from build123d import *

# Parameters (mm, degrees)
F0_W           = 50.8
F0_H           = 38.1
F1_DEPTH       = 3.175
F3_START       = -18.288
F2_W           = 38.1
F2_H           = 69.85
F3_DEPTH       = 3.556
F5_START       = 27.686
F4_W           = 38.1
F4_H           = 69.85
F5_DEPTH       = 3.81
F6_W           = 19.05
F6_H           = 53.975
F7_DEPTH       = 32.004
F8_T1_DEPTH    = 64.9044340938
F8_T3_DEPTH    = 19.05
F8_T5_DEPTH    = 62.6934442484
F8_T11_DEPTH   = 64.9044340938
F8_T15_DEPTH   = 31.165027858
F8_T23_DEPTH   = 31.165027858
F8_T28_DEPTH   = 64.9044340938
F9_W           = 54.9304988235
F9_H           = 1.4888443984
F10_DEPTH      = 28.4988
F10_DEPTH_BACK = 25.4


# Not quite as in the source:
# - a fillet or chamfer that OpenCascade refuses, or shapes differently, is made with other operations: its cross-section is extruded or revolved along the edge and cut away or added


with BuildPart() as f1:
    # F0 (on Top) → F1 (new body)
    with BuildSketch(Plane.XY):
        with Locations((3.5055922344, 6.6658267866)):
            Rectangle(F0_W, F0_H)
    extrude(amount=F1_DEPTH)

    # F2 (on Right) → F3 (join)
    with BuildSketch(Plane.YZ.offset(F3_START)):
        with Locations((6.8596902806, -32.1689685807)):
            Rectangle(F2_W, F2_H)
    extrude(amount=-F3_DEPTH)

    # F4 (on Right) → F5 (join)
    with BuildSketch(Plane.YZ.offset(F5_START)):
        with Locations((7.2173965164, -31.5503366292)):
            Rectangle(F4_W, F4_H)
    extrude(amount=F5_DEPTH)

    # F6 (on Right) → F7 (cut)
    with BuildSketch(Plane.YZ):
        with Locations((6.4956571441, -41.2920623448)):
            Rectangle(F6_W, F6_H)
    extrude(amount=-F7_DEPTH, mode=Mode.SUBTRACT)

    # F8: fillet of radius 5.08 on 4 edges, made by hand

    # F8_s2 → F8_t1 (cut)
    with BuildSketch(Plane.XY.offset(-79.2089964387)):
        with BuildLine():
            ThreePointArc((-18.288, 20.8666682873), (-19.2723730639, 17.8612997575), (-21.844, 16.0206571441))
            Line((-21.844, 16.0206571441), (-18.288, 16.0206571441))
            Line((-18.288, 16.0206571441), (-18.288, 20.8666682873))
        make_face()
        with BuildLine():
            ThreePointArc((-18.288, -7.8753539991), (-19.2723730639, -4.8699854693), (-21.844, -3.0293428559))
            Line((-21.844, -3.0293428559), (-18.288, -3.0293428559))
            Line((-18.288, -3.0293428559), (-18.288, -7.8753539991))
        make_face()
    extrude(amount=F8_T1_DEPTH, mode=Mode.SUBTRACT)

    # F8_s4 → F8_t3 (cut)
    with BuildSketch(Plane.XZ.offset(-16.0206571441)):
        with BuildLine():
            ThreePointArc((-18.288, -9.4585512016), (-19.2723730639, -12.4639197314), (-21.844, -14.3045623448))
            Line((-21.844, -14.3045623448), (-18.288, -14.3045623448))
            Line((-18.288, -14.3045623448), (-18.288, -9.4585512016))
        make_face()
    extrude(amount=F8_T3_DEPTH, mode=Mode.SUBTRACT)

    # F8_s6 → F8_t5 (cut)
    with BuildSketch(Plane.XZ.offset(-38.5641186406)):
        with BuildLine():
            ThreePointArc((27.686, -61.5566477795), (28.7499073716, -64.6674997528), (31.496, -66.4753366292))
            Line((31.496, -66.4753366292), (27.686, -66.4753366292))
            Line((27.686, -66.4753366292), (27.686, -61.5566477795))
        make_face()
    extrude(amount=F8_T5_DEPTH, mode=Mode.SUBTRACT)


with BuildPart() as f8_tool9:
    # F8_s10 → F8_t11 (new body)
    with BuildSketch(Plane.XY.offset(-67.0939685807)):
        with BuildLine():
            ThreePointArc((-18.288, 20.8666682873), (-19.2723730639, 17.8612997575), (-21.844, 16.0206571441))
            Line((-21.844, 16.0206571441), (-18.288, 16.0206571441))
            Line((-18.288, 16.0206571441), (-18.288, 20.8666682873))
        make_face()
    extrude(amount=F8_T11_DEPTH)

    split(bisect_by=Plane.XY.offset(-14.3045623448), keep=Keep.TOP)


with BuildPart() as f8_tool13:
    # F8_s14 → F8_t15 (new body)
    with BuildSketch(Plane.XZ.offset(-28.1356850021)):
        with BuildLine():
            ThreePointArc((-18.288, -9.4585512016), (-19.2723730639, -12.4639197314), (-21.844, -14.3045623448))
            Line((-21.844, -14.3045623448), (-18.288, -14.3045623448))
            Line((-18.288, -14.3045623448), (-18.288, -9.4585512016))
        make_face()
    extrude(amount=F8_T15_DEPTH)

    split(bisect_by=Plane.XZ.offset(-25.9096902806), keep=Keep.TOP)

    split(bisect_by=Plane.XZ.offset(-16.0206571441), keep=Keep.BOTTOM)


with BuildPart() as f8_tool9_1:
    add(f8_tool9.part)

    # F8_t18: intersect F8_tool13
    add(f8_tool13.part, mode=Mode.INTERSECT)


with BuildPart() as f1_1:
    add(f1.part)

    # F8_t7: cut F8_tool9
    add(f8_tool9_1.part, mode=Mode.SUBTRACT)


with BuildPart() as f8_tool21:
    # F8_s22 → F8_t23 (new body)
    with BuildSketch(Plane.XZ.offset(-16.0206571441)):
        with BuildLine():
            ThreePointArc((-18.288, -9.4585512016), (-19.2723730639, -12.4639197314), (-21.844, -14.3045623448))
            Line((-21.844, -14.3045623448), (-18.288, -14.3045623448))
            Line((-18.288, -14.3045623448), (-18.288, -9.4585512016))
        make_face()
    extrude(amount=F8_T23_DEPTH)

    split(bisect_by=Plane.XZ.offset(12.1903097194), keep=Keep.BOTTOM)

    split(bisect_by=Plane.XZ.offset(3.0293428559), keep=Keep.TOP)


with BuildPart() as f8_tool26:
    # F8_s27 → F8_t28 (new body)
    with BuildSketch(Plane.XY.offset(-2.1895344868)):
        with BuildLine():
            ThreePointArc((-18.288, -7.8753539991), (-19.2723730639, -4.8699854693), (-21.844, -3.0293428559))
            Line((-21.844, -3.0293428559), (-18.288, -3.0293428559))
            Line((-18.288, -3.0293428559), (-18.288, -7.8753539991))
        make_face()
    extrude(amount=-F8_T28_DEPTH)

    split(bisect_by=Plane.XY.offset(-14.3045623448), keep=Keep.TOP)


with BuildPart() as f8_tool21_1:
    add(f8_tool21.part)

    # F8_t30: intersect F8_tool26
    add(f8_tool26.part, mode=Mode.INTERSECT)


with BuildPart() as f1_2:
    add(f1_1.part)

    # F8_t19: cut F8_tool21
    add(f8_tool21_1.part, mode=Mode.SUBTRACT)

    # F9 (on Front) → F10 (cut, two sides)
    with BuildSketch(Plane.XZ) as f10_sk:
        with Locations((4.6410532668, 3.4134599846)):
            Rectangle(F9_W, F9_H)
    extrude(amount=-F10_DEPTH, mode=Mode.SUBTRACT)
    extrude(f10_sk.sketch, amount=F10_DEPTH_BACK, mode=Mode.SUBTRACT)


solid = f1_2.part
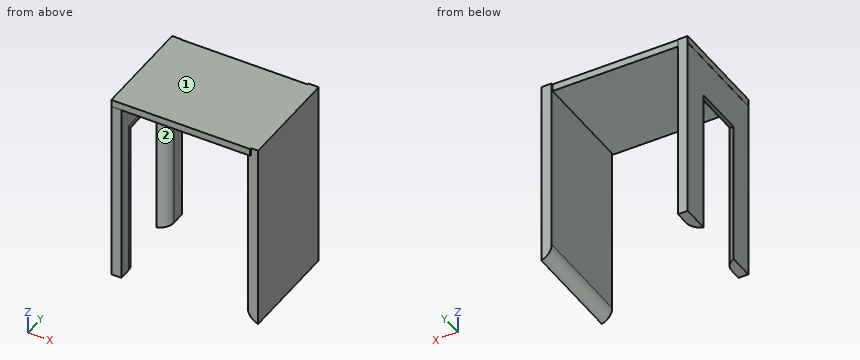
CAD build for the part. Positions are in the model's coordinates, mm. Face numbers are marked on the shaded views. Give positions to 0.01 mm unless a question says otherwise; leave off trailing zeros. Write each loop counter-clockwise with the first axis right and the second up, starting at its lowest first coordinate (ties: lowest second). Pieces come first, ordered by that corner, then holes. Notation, with made-up numbers: M 6.5,46.5 L 10.5,46.5 A23 cw 10.5,58.5 Z; hole C -13.5,61.25 d1. An arc over 180 degrees is marked long. Put each result on its own line as item: value. Start each with the question number.
(1) Band-saw the part on D-D, the plane x = -10.5. Write the cut outline in (y, z), and give its area (3 significant figures).
(2) Band-saw the part on B-B, the plane z = -38.5. Write the cut outline in (x, y).
(3) Band-saw the part on C-C, the plane y = 14. Write the cut outline in (x, z).
(4) Band-saw the part on A-A, the plane z = -2. Write the cut outline in (x, y).
(5) Probe L1, parallel to X at y = 18, z = -5; L2, parallel to X at y = 13, z = -51; L3, parallel to Z at x = -13, y = 15.5. List the from-to ranges inside material, lowest first.
(6) Mould opens along Y. For the marked faces 1 and 2 say: +Y half, -Y half, draft (parallel to the pull), parting line (faces both ways), or undercut.
(7) Flat gauge pins, fed straight in: pin 1 Ø8 at (x, z) = (-15, -32) entering from -Y; pin 2 Ø3 at (x, z) = (29.5, -15) entering from -Y; pin 3 Ø12 at (x, z) = (20, -4.5) entering from +Y. Where does each tip first touch, or does it go through?
Response values:
1. outline: M -12.38,0 L 25.72,0 L 25.72,2.67 L -12.38,2.67 Z
1. area: 102 mm2
2. outline: M -21.84,-12.19 L -18.29,-12.19 L -18.29,-7.88 A5.08 ccw -21.84,-3.03 Z; M -21.84,16.02 A5.08 ccw -18.29,20.87 L -18.29,25.91 L -21.84,25.91 Z; M 27.69,-11.83 L 31.5,-11.83 L 31.5,26.27 L 27.69,26.27 Z
3. outline: M -21.89,0 L -21.84,0 L -21.84,-14.3 A5.08 ccw -18.29,-9.46 L -18.29,0 L 27.69,0 L 27.69,-61.56 A5.08 ccw 31.5,-66.48 L 31.5,2.67 L -21.89,2.67 Z
4. outline: M -21.84,-12.19 L -18.29,-12.19 L -18.29,25.91 L -21.84,25.91 Z; M 27.69,-11.83 L 31.5,-11.83 L 31.5,26.27 L 27.69,26.27 Z
5. L1: x = -21.84 to -18.29, 27.69 to 31.5
5. L2: x = 27.69 to 31.5
5. L3: z = 0 to 2.67
6. face 1: draft
6. face 2: undercut
7. pin 1: stops at y = -12.19
7. pin 2: stops at y = -11.83
7. pin 3: stops at y = 25.72
